```python
from build123d import *

# Parameters (mm, degrees)
SKETCH2_W     = 38.1
SKETCH2_H     = 10.31875
SKETCH2_W_2   = 23.8125
SKETCH2_H_2   = 9.525
CHAMFER4_SIZE = 1.5875
CHAMFER5_SIZE = 1.5875
SKETCH3_W     = 4.7625
SKETCH3_H     = 4.7625


with BuildPart() as part:
    # Sketch2 → Revolve1 (revolve)
    with BuildSketch(Plane.XY):
        Polygon((-90.4875, 12.7), (-90.4875, 0), (-66.675, 0), (-66.675, 11.1125), (-66.675, 12.7), align=None)
        Polygon((-66.675, 11.1125), (-66.675, 0), (-38.1, 0), (-38.1, 10.31875), (-38.1, 11.1125), align=None)
        with Locations((-19.05, 5.159375)):
            Rectangle(SKETCH2_W, SKETCH2_H)
        with Locations((19.05, 5.159375)):
            Rectangle(SKETCH2_W, SKETCH2_H)
        Polygon((38.1, 10.31875), (38.1, 0), (66.675, 0), (66.675, 9.525), (66.675, 11.1125), (38.1, 11.1125), align=None)
        with Locations((78.58125, 4.7625)):
            Rectangle(SKETCH2_W_2, SKETCH2_H_2)
    revolve(axis=Axis((90.4875, 0, 0), (-1, 0, 0)))

    # Chamfer4
    chamfer4_edges = [part.edges().sort_by_distance(p)[0] for p in [
        (90.4875, -9.525, 0),
    ]]
    chamfer(chamfer4_edges, length=CHAMFER4_SIZE)

    # Chamfer5
    chamfer5_edges = [part.edges().sort_by_distance(p)[0] for p in [
        (-90.4875, -12.7, 0),
    ]]
    chamfer(chamfer5_edges, length=CHAMFER5_SIZE)

    # Sketch3 → Cut-Revolve1 (revolve, cut)
    with BuildSketch(Plane.XY, mode=Mode.PRIVATE) as cut_revolve1_sk:
        with Locations((-54.76875, -8.73125)):
            Rectangle(SKETCH3_W, SKETCH3_H)
    revolve(cut_revolve1_sk.sketch.rotate(Axis((-52.3875, -1001.138899493, 0), (0, 1, 0)), 270), axis=Axis((-52.3875, -1001.138899493, 0), (0, 1, 0)), mode=Mode.SUBTRACT)


solid = part.part
```
Geometry: final body of the model. Coordinates: model frame, mm. A direction names the side the tool comes from. Round coordinates to 2 decimals unless told otherwise and drop trailing zeros. Write each loop counter-clockwise with the first axis right and the second up, starting at its lowest first coordinate (ties: lowest second). Pieces come first, ordered by that corner, then holes. Notation, with made-up numbers: M 16,49.5 L 29,49.5 A15 cw 29,60.5 Z; hole C 62.25,-6.75 d5. An arc over 180 degrees is marked long. Answer in a Markdown table with one row per item. Add a question column.
(1) Contact query for flat-ended pins moving along their axis: pin 1 (1 mm diameter, centred on y = -3, z = -10, fed in from +X) (3 decimals); pin 2 (10 mm diameter, centred on x = 25.5, y = 7.5, fed in from -Z); pin 3 (1 mm diameter, centred on x = 68.5, y = -5, fed in from -Z) (3 decimals). Output: stop coordinate, or through.
(2) Cut plane D-D, the plane x = 62. Return the cut outline in (y, z) (1 decimal), then the cut area to 3 significant figures.
(3) Draft query along Z for faces 1 (the face through (-90.488, 0, 0)), 2 (the face through (77.943, -7.559, 5.796)), 3 (the face through (-52, -6.35, 0)), 4 (the face through (-49.49, -8.7, 3.78)). Return one class per face: pulls with the +Z half, pulls with the -Z half, needs draft (parallel to the pull), parting line crosses it, or undercut.
(4) Ray query, L1, parallel to X at y = -5.75, z = 9 (1 decimal); L2, parallel to Y at x = -56.5, z = 0; L3, parallel to Z at x = -56, y = -7.5. Return the intervals inside material, ascending.
(5) Cut plane C-C, the plane x = -28. Return the cut outline in (y, z), then the cut area to 3 significant figures.
(6) Reachability of faces 5 (the face through (-38.1, -7, 8)), 6 (the face through (66.675, 5, -8.3)), 7 (the face through (90.488, 0, 0)) from +Z, -Z, +X, -X, +Y, -Y: full face, straight path, thin tool, end or side. Return the list, or none.
(7) Cut plane A-A, the plane y = 0. Return the cut outline in (x, z) (1 decimal), then the cut area to 3 significant figures.
Established:
| question | item | result |
|---|---|---|
| 1 | pin 1 | x = 66.675 |
| 1 | pin 2 | z = -10.01 |
| 1 | pin 3 | z = -8.395 |
| 2 | outline | C 0,0 d22.2 |
| 2 | area | 388 mm² |
| 3 | face 1 | needs draft |
| 3 | face 2 | parting line crosses it |
| 3 | face 3 | undercut |
| 3 | face 4 | undercut |
| 4 | L1 | -90.5 to -38.1, 38.1 to 66.7 |
| 4 | L2 | -6.35 to 11.11 |
| 4 | L3 | -8.2 to -3.1, 3.1 to 8.2 |
| 5 | outline | C 0,0 d20.64 |
| 5 | area | 335 mm² |
| 6 | face 5 | none |
| 6 | face 6 | +X |
| 6 | face 7 | +Z, -Z, +X, +Y, -Y |
| 7 | outline | M -90.5,-11.1 L -88.9,-12.7 L -66.7,-12.7 L -66.7,-11.1 L -38.1,-11.1 L -38.1,-10.3 L 38.1,-10.3 L 38.1,-11.1 L 66.7,-11.1 L 66.7,-9.5 L 88.9,-9.5 L 90.5,-7.9 L 90.5,7.9 L 88.9,9.5 L 66.7,9.5 L 66.7,11.1 L 38.1,11.1 L 38.1,10.3 L -38.1,10.3 L -38.1,11.1 L -66.7,11.1 L -66.7,12.7 L -88.9,12.7 L -90.5,11.1 Z |
| 7 | area | 3,900 mm² |
